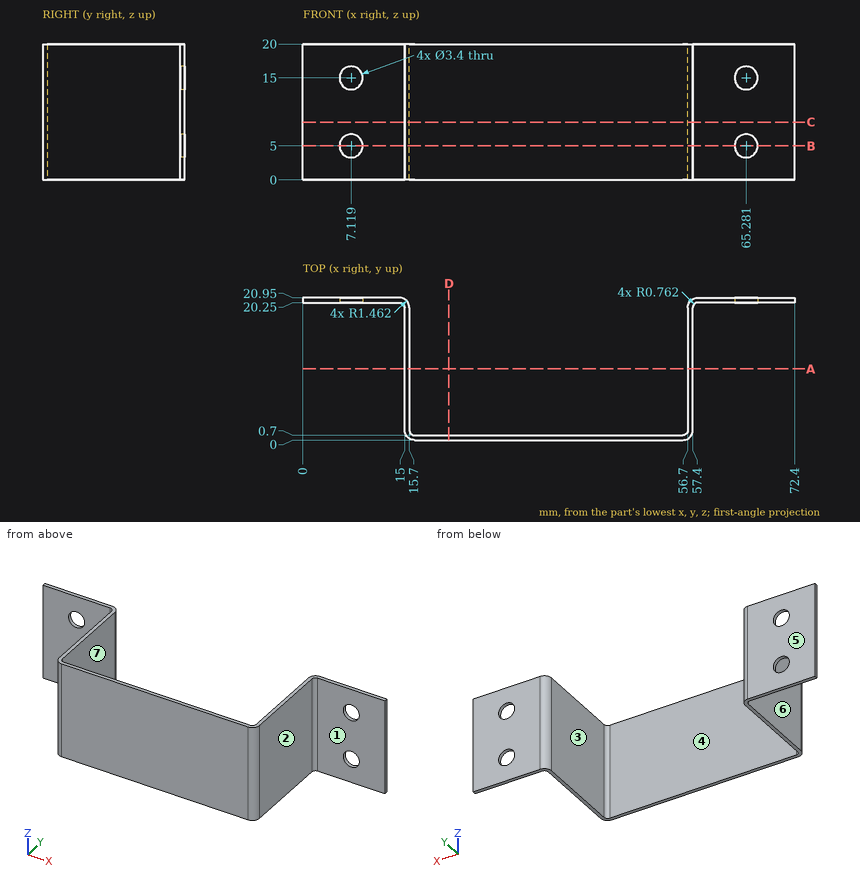
Geometry check sheet. Reference: drawing and pictorial views, mm from the part's lowest x, y, z. A direction names the side the tool comes from. Coordinates: 2 decimals unless noted, no trailing zeros. Order: outer loops, then holes, each group sorted by start corner. A loop starts at its lowest first (then second) coordinate and runs counter-clockwise, first axis right, second up. Notation, with made-up numbers: (70.25, 56) -> (122.25, 56) arc R9 cw to (122.25, 72) -> close; hole circle Ø5 at (6, 64). An arc over 180 degrees is marked (long way). Use CSV: the item, a comma, the result in double quotes. Start each with the question number.
Q1. Section check A-A, the plane y = 10.5. Record the cut outline in (x, z), and give its area (3 significant figures).
Q2. Draft check along X on the marked faces 1, 2, 3 and 4. Enter one of: +X half, -X half, draft (parallel to the pull), parting line (faces both ways), or undercut.
Q3. Depth check by flat-ended pin: P1, Ø5, axis at x = 60, y = 11.5, coming from the +Z side; P2, Ø11.5, axis at x = 9.5, z = 5.5, coming from the -Y side; P3, Ø5.5, axis at y = 7, z = 9, coming from the -X side; P4, Ø5.5, axis at x = 7.119, z = 15, coming from the -Y side. Enter the tip coordinate at first touch or a pass-through.
Q4. Section check D-D, the plane x = 21.5. Record the cut outline in (y, z).
Q5. Section check C-C, the plane z = 8.5. Record the cut outline in (x, y), and give its area (3 significant figures).
Q6. Thickness scan on line 1 along X through (y, z) = (12.5, 15.5); line 2 along X through (y, z) = (20.6, 15); line 3 along X through (y, z) = (20.7, 15). Record the ranges inside material, lowest first.
Q7. Tool access check on the marked faces 5, 6 and 7. Record the directions out of +Z, -Z, +X, -X, +Y, -Y that give a thin tool (end or side, any length) a straight path to the whole face; none if there is none.
Q8. Section check B-B, the plane z = 5. Record the cut outline in (x, y), and give its area (3 significant figures).
Returned:
1,outline,"(15, 0) -> (15.7, 0) -> (15.7, 20) -> (15, 20) -> close; (56.7, 0) -> (57.4, 0) -> (57.4, 20) -> (56.7, 20) -> close"
1,area,"28.0 mm^2"
2,face 1,"draft"
2,face 2,"+X half"
2,face 3,"undercut"
2,face 4,"undercut"
3,P1,"passes through"
3,P2,"stops at y = 0.64"
3,P3,"stops at x = 15"
3,P4,"stops at y = 20.25"
4,outline,"(0, 0) -> (0.7, 0) -> (0.7, 20) -> (0, 20) -> close"
5,outline,"(0, 20.25) -> (14.24, 20.25) arc R0.76 cw to (15, 19.49) -> (15, 1.46) arc R1.46 ccw to (16.46, 0) -> (55.94, 0) arc R1.46 ccw to (57.4, 1.46) -> (57.4, 19.49) arc R0.76 cw to (58.16, 20.25) -> (72.4, 20.25) -> (72.4, 20.95) -> (58.16, 20.95) arc R1.46 ccw to (56.7, 19.49) -> (56.7, 1.46) arc R0.76 cw to (55.94, 0.7) -> (16.46, 0.7) arc R0.76 cw to (15.7, 1.46) -> (15.7, 19.49) arc R1.46 ccw to (14.24, 20.95) -> (0, 20.95) -> close"
5,area,"77.7 mm^2"
6,line 1,"x = 15 to 15.7, 56.7 to 57.4"
6,line 2,"x = 0 to 5.42, 8.82 to 15.19, 57.21 to 63.58, 66.98 to 72.4"
6,line 3,"x = 0 to 5.42, 8.82 to 15.06, 57.34 to 63.58, 66.98 to 72.4"
7,face 5,"+Z, -Z, +X, -X, +Y"
7,face 6,"+Z, -Z, -X, -Y"
7,face 7,"+Z, -Z, +Y"
8,outline,"(0, 20.25) -> (5.42, 20.25) -> (5.42, 20.95) -> (0, 20.95) -> close; (8.82, 20.25) -> (14.24, 20.25) arc R0.76 cw to (15, 19.49) -> (15, 1.46) arc R1.46 ccw to (16.46, 0) -> (55.94, 0) arc R1.46 ccw to (57.4, 1.46) -> (57.4, 19.49) arc R0.76 cw to (58.16, 20.25) -> (63.58, 20.25) -> (63.58, 20.95) -> (58.16, 20.95) arc R1.46 ccw to (56.7, 19.49) -> (56.7, 1.46) arc R0.76 cw to (55.94, 0.7) -> (16.46, 0.7) arc R0.76 cw to (15.7, 1.46) -> (15.7, 19.49) arc R1.46 ccw to (14.24, 20.95) -> (8.82, 20.95) -> close; (66.98, 20.25) -> (72.4, 20.25) -> (72.4, 20.95) -> (66.98, 20.95) -> close"
8,area,"72.9 mm^2"
